from build123d import *
from build123d.topology import SkipClean

# Parameters (mm, degrees)
SKETCH1_R           = 5.35
BOSS_EXTRUDE1_DEPTH = 2.5
HOLE1_OUTLINE_R     = 1.7
HOLE1_DEPTH         = 2.5
SKETCH3_R           = 3
SKETCH3_R_2         = 1.7
BOSS_EXTRUDE2_DEPTH = 10
FILLET1_R           = 0.1
BOSS_EXTRUDE3_DEPTH = 1.5
SKETCH8_R           = 0.75
CUT_EXTRUDE1_DEPTH  = 13.539736839
CUT_EXTRUDE3_START  = -0.5
SKETCH13_R          = 1.25
CUT_EXTRUDE3_DEPTH  = 7
CHAMFER1_SIZE       = 0.25
CUT_EXTRUDE4_START  = -0.5
CUT_EXTRUDE4_DEPTH  = 0.5
FILLET2_R           = 0.4


# Read off the part's stored shape, not the designer's step: Hole1
with BuildPart() as part:
    # Sketch1 → Boss-Extrude1 (new body)
    with BuildSketch(Plane(origin=(0, 0, 0), x_dir=(1, 0, 0), z_dir=(0, 1, 0))):
        with Locations(Location((0, 0, 0), (0, 0, 270))):
            Circle(SKETCH1_R)
    extrude(amount=BOSS_EXTRUDE1_DEPTH)

    # Hole1 outline → Hole1 (cut)
    with BuildSketch(Plane(origin=(0, 0, 0), x_dir=(1, 0, 0), z_dir=(0, 1, 0))):
        Circle(HOLE1_OUTLINE_R)
    extrude(amount=HOLE1_DEPTH, mode=Mode.SUBTRACT)

    # Sketch3 → Boss-Extrude2 (add)
    with BuildSketch(Plane(origin=(0, 2.5, 0), x_dir=(1, 0, 0), z_dir=(0, 1, 0))):
        with Locations(Location((0, 0, 0), (0, 0, 270))):
            Circle(SKETCH3_R)
        with Locations(Location((0, 0, 0), (0, 0, 270))):
            Circle(SKETCH3_R_2, mode=Mode.SUBTRACT)
    extrude(amount=BOSS_EXTRUDE2_DEPTH)

    # Fillet1
    fillet1_edges = [part.edges().sort_by_distance(p)[0] for p in [
        (0, 12.5, -3),
    ]]
    fillet(fillet1_edges, radius=FILLET1_R)

    # Sketch5 → Boss-Extrude3 (add)
    with BuildSketch(Plane(origin=(0, 2.5, 0), x_dir=(1, 0, 0), z_dir=(0, 1, 0))):
        with BuildLine():
            Line((-0.75, 5.297169055), (-0.75, 2.90473751))
            ThreePointArc((-0.75, 2.90473751), (0, 3), (0.75, 2.90473751))
            Line((0.75, 2.90473751), (0.75, 5.297169055))
            ThreePointArc((0.75, 5.297169055), (0, 5.35), (-0.75, 5.297169055))
        make_face()
    boss_extrude3 = extrude(amount=BOSS_EXTRUDE3_DEPTH)

    # Mirror1: Boss-Extrude3 across plane
    with SkipClean():  # the faces are left unmerged after this step: merging them gives an invalid solid
        add(boss_extrude3.mirror(Plane.XY))

    # Sketch8 → Cut-Extrude1 (cut, through all)
    with SkipClean():  # the faces are left unmerged after this step: merging them gives an invalid solid
        with BuildSketch(Plane(origin=(0, 2.5, 0), x_dir=(1, 0, 0), z_dir=(0, 1, 0))):
            with Locations(Location((3.8, 0, 0), (0, 0, 270))):
                Circle(SKETCH8_R)
            with Locations(Location((-1.9, -3.290896534, 0), (0, 0, 270))):
                Circle(SKETCH8_R)
            with Locations(Location((-1.9, 3.290896534, 0), (0, 0, 270))):
                Circle(SKETCH8_R)
        extrude(amount=-CUT_EXTRUDE1_DEPTH, mode=Mode.SUBTRACT)

    # Sketch13 → Cut-Extrude3 (cut)
    with SkipClean():  # the faces are left unmerged after this step: merging them gives an invalid solid
        with BuildSketch(Plane(origin=(0, 2.5, 0), x_dir=(1, 0, 0), z_dir=(0, 1, 0)).offset(CUT_EXTRUDE3_START)):
            with Locations(Location((-1.9, 3.290896534, 0), (0, 0, 23.073918066))):
                Circle(SKETCH13_R)
            with Locations(Location((-1.9, -3.290896534, 0), (0, 0, 102.514591278))):
                Circle(SKETCH13_R)
            with Locations(Location((3.8, 0, 0), (0, 0, 137.485408722))):
                Circle(SKETCH13_R)
        extrude(amount=CUT_EXTRUDE3_DEPTH, mode=Mode.SUBTRACT)

    # Chamfer1
    chamfer1_edges = [part.edges().sort_by_distance(p)[0] for p in [
        (-1.275, 9, -2.20836478),
        (-1.275, 9, 2.20836478),
        (2.55, 9, 0),
    ]]
    chamfer(chamfer1_edges, length=CHAMFER1_SIZE)

    # Sketch14 → Cut-Extrude4 (cut)
    with BuildSketch(Plane(origin=(0, 2.5, 0), x_dir=(1, 0, 0), z_dir=(0, 1, 0)).offset(CUT_EXTRUDE4_START)):
        with BuildLine():
            Line((-0.75, -3.780794483), (-0.75, -5.297169055))
            ThreePointArc((-0.75, -5.297169055), (-2.563606422, -4.695787699), (-4.050222345, -3.495454041))
            Line((-4.050222345, -3.495454041), (-2.716694869, -2.344582902))
            ThreePointArc((-2.716694869, -2.344582902), (-2.637189937, -4.300377092), (-0.75, -3.780794483))
        make_face()
        with BuildLine():
            Line((-0.75, 5.297169055), (-0.75, 3.780794483))
            ThreePointArc((-0.75, 3.780794483), (-2.637189937, 4.300377092), (-2.716694869, 2.344582902))
            Line((-2.716694869, 2.344582902), (-4.050222345, 3.495454041))
            ThreePointArc((-4.050222345, 3.495454041), (-2.563606422, 4.695787699), (-0.75, 5.297169055))
        make_face()
        with BuildLine():
            Line((3.388815789, -1.18043532), (5.05226317, -1.759868421))
            ThreePointArc((5.05226317, -1.759868421), (5.35, 0), (5.05226317, 1.759868421))
            Line((5.05226317, 1.759868421), (3.388815789, 1.18043532))
            ThreePointArc((3.388815789, 1.18043532), (5.05, 0), (3.388815789, -1.18043532))
        make_face()
    extrude(amount=CUT_EXTRUDE4_DEPTH, mode=Mode.SUBTRACT)

    # Fillet2
    fillet2_edges = [part.edges().sort_by_distance(p)[0] for p in [
        (-4.050222345, 2.25, -3.495454041),
        (-4.050222345, 2.25, 3.495454041),
        (5.05226317, 2.25, -1.759868421),
        (5.05226317, 2.25, 1.759868421),
    ]]
    fillet(fillet2_edges, radius=FILLET2_R)


solid = part.part
The listing builds one solid part. Answer for the finished solid, in the listing's coordinates (mm). A direction names the side the tool comes from. Coordinates: 2 decimals unless noted, no trailing zeros. Write each loop counter-clockwise with the first axis right and the second up, starting at its lowest first coordinate (ties: lowest second). Pieces come first, ordered by that corner, then holes. Notation, with made-up numbers: (-19.75, 68) -> (30.25, 68) arc R20 ccw to (30.25, 86) -> close; hole circle Ø2 at (57.5, 71.5). An arc over 180 degrees is marked (long way). One line per question, with ' | ' between items.
1. Section B-B (x = 0) is taken. Determine the outline of the cut face in (y, z).
Verdict:
outline: (0, -5.35) -> (4, -5.35) -> (4, -3) -> (12.4, -3) arc R0.1 ccw to (12.5, -2.9) -> (12.5, -1.7) -> (0, -1.7) -> close; (0, 1.7) -> (12.5, 1.7) -> (12.5, 2.9) arc R0.1 ccw to (12.4, 3) -> (4, 3) -> (4, 5.35) -> (0, 5.35) -> close
2. Straight lines are drawn through the part: line 1 (Y direction, x = -2.25, z = 2.5); line 2 (X direction, y = 10, z = 0); line 3 (Y direction, x = -2.75, z = -2.25). For each, find the intervals that lie inside material, in ascending order.
Verdict:
line 1: y = 0 to 2 | line 2: x = -3 to -1.7, 1.7 to 3 | line 3: y = 0 to 2.5
3. For a pull along Y with two mould halves and no side action, classify faces 1 (the cylindrical face through (-1.675, 1.014, -2.576)), 2 (the flat face through (0, 0, 2)), 3 (the flat face through (5, 2, -1)) as released by +Y, released by -Y, zero draft, split by the parting line, or undercut.
Verdict:
face 1: zero draft | face 2: released by -Y | face 3: undercut
4. Section C-C (z = 0) is taken. Determine the outline of the cut face in (x, y).
Verdict:
outline: (-5.35, 0) -> (-1.7, 0) -> (-1.7, 12.5) -> (-2.9, 12.5) arc R0.1 ccw to (-3, 12.4) -> (-3, 2.5) -> (-5.35, 2.5) -> close; (1.7, 0) -> (3.05, 0) -> (3.05, 2) -> (2.55, 2) -> (2.55, 8.75) -> (2.8, 9) -> (3, 9) -> (3, 12.4) arc R0.1 ccw to (2.9, 12.5) -> (1.7, 12.5) -> close; (4.55, 0) -> (5.35, 0) -> (5.35, 2) -> (4.55, 2) -> close
5. Which of the six approach directions +Z, -Z, +X, -X, +Y, -Y give full straight-line access (tool end or side, diameter ignored) to faces 4 (the flat face through (-3.23, 2.25, 2.79)), 5 (the flat face through (-3.22, 2.25, -2.78)), 6 (the cylindrical face through (0.9, 8.48, 2.86)), 7 (the flat face through (-0.75, 3, -5))?
Verdict:
face 4: +Z, +Y | face 5: -Z, +Y | face 6: +Y | face 7: -Z, -X, +Y
6. Section A-A (y = 1.75) is taken. Determine the outline of the cut face in (x, z), and give its area (3 significant figures).
Verdict:
outline: circle Ø10.7 at (0, 0); hole circle Ø1.5 at (-1.9, -3.29); hole circle Ø1.5 at (-1.9, 3.29); hole circle Ø3.4 at (0, 0); hole circle Ø1.5 at (3.8, 0) | area: 75.5 mm^2
7. Given pin 1 Ø1.7 at (y, z) = (3.5, -4) entering from -X; pin 2 Ø1.2 at (x, z) = (0, 4.5) entering from +Y; pin 3 Ø1.3 at (x, z) = (2, 3.5) entering from +Y, each flat-ended and moving along its own axis, determine where each tip first touches the part or whether it passes through.
Verdict:
pin 1: stops at x = -0.75 | pin 2: stops at y = 4 | pin 3: stops at y = 2.5
8. Section D-D (y = 5.75) is taken. Determine the outline of the cut face in (x, z).
Verdict:
outline: (-2.17, -2.07) arc R1.25 cw to (-0.71, -2.92) arc R3 ccw to (2.88, -0.84) arc R1.25 cw to (2.88, 0.84) arc R3 ccw to (-0.71, 2.92) arc R1.25 cw to (-2.17, 2.07) arc R3 ccw to start; hole circle Ø3.4 at (0, 0)
